Autodesk Inventor part; units mm, degrees
ref_plane "YZ Plane" through (0, 0, 0) normal (1, 0, 0) x (0, 1, 0)
ref_plane "XZ Plane" through (0, 0, 0) normal (0, 1, 0) x (-1, 0, 0)
ref_plane "XY Plane" through (0, 0, 0) normal (0, 0, 1) x (1, 0, 0)
sketch "スケッチ5" plane through (0, 0, 0) normal (1, 0, 0) x (0, 1, 0)
  circle A0 centre (68.5779, -0.3457) radius 120
  line L0 (68.5779, -0.3457) -> (-262.8846, -0.3457) construction
  line L1 (136.0779, -117.2592) -> (-66.4221, -0.3457)
  circle A1 centre (68.5779, -0.3457) radius 5
  line L2 (68.5779, -0.3457) -> (136.0779, 116.5677) construction
  line L3 (68.5779, -0.3457) -> (136.0779, -117.2592) construction
  line L4 (68.5779, -0.3457) -> (-66.4221, -0.3457)
  line L5 (85.6138, 37.1613) -> (80.6138, 28.5011) construction
  line L6 (80.6138, 28.5011) -> (84.0779, 26.5011) construction
  line L7 (84.0779, 26.5011) -> (89.0779, 35.1613) construction
  line L8 (89.0779, 35.1613) -> (85.6138, 37.1613)
  line L9 (89.0779, 35.1613) -> (84.0779, 26.5011) construction
  line L10 (84.0779, 26.5011) -> (87.542, 24.5011) construction
  line L11 (87.542, 24.5011) -> (92.542, 33.1613) construction
  line L12 (92.542, 33.1613) -> (89.0779, 35.1613)
  line L13 (83.1138, 32.8312) -> (90.042, 28.8312) construction
  circle A2 centre (68.5779, -0.3457) radius 2.65 construction
  line L14 (85.3973, 37.2863) -> (78.8973, 26.028) construction
  line L15 (78.8973, 26.028) -> (74.5672, 28.528) construction
  line L16 (74.5672, 28.528) -> (81.0672, 39.7863) construction
  line L17 (81.0672, 39.7863) -> (85.3973, 37.2863)
  line L18 (92.7585, 33.0363) -> (86.2585, 21.778) construction
  line L19 (86.2585, 21.778) -> (90.5886, 19.278) construction
  line L20 (90.5886, 19.278) -> (97.0886, 30.5363) construction
  line L21 (97.0886, 30.5363) -> (92.7585, 33.0363)
  circle A3 centre (68.5779, -0.3457) radius 28.3207 construction
  line L22 (27.5779, 8.9043) -> (27.5779, 3.9043)
  line L23 (27.5779, 3.9043) -> (40.5779, 3.9043) construction
  line L24 (40.5779, 8.9043) -> (27.5779, 8.9043) construction
  line L25 (40.5779, 3.9043) -> (40.5779, 8.9043)
  line L26 (27.5779, -4.5957) -> (40.5779, -4.5957) construction
  line L27 (27.5779, -9.5957) -> (27.5779, -4.5957)
  line L28 (40.5779, -9.5957) -> (27.5779, -9.5957) construction
  line L29 (40.5779, -4.5957) -> (40.5779, -9.5957)
  line L30 (81.0672, -40.4778) -> (85.3973, -37.9778)
  line L31 (85.3973, -37.9778) -> (78.8973, -26.7194) construction
  line L32 (74.5672, -29.2194) -> (81.0672, -40.4778) construction
  line L33 (78.8973, -26.7194) -> (74.5672, -29.2194) construction
  line L34 (92.7585, -33.7278) -> (86.2585, -22.4694) construction
  line L35 (97.0886, -31.2278) -> (92.7585, -33.7278)
  line L36 (90.5886, -19.9694) -> (97.0886, -31.2278) construction
  line L37 (86.2585, -22.4694) -> (90.5886, -19.9694) construction
  line L38 (74.5672, 28.528) -> (73.9509, 27.4606)
  line L39 (90.5886, 19.278) -> (89.9724, 18.2106) construction
  line L40 (40.5779, 8.9043) -> (41.8104, 8.9043)
  line L41 (40.5779, -9.5957) -> (41.8104, -9.5957)
  line L42 (74.5672, -29.2194) -> (70.7713, -22.6449)
  line L43 (90.5886, -19.9694) -> (89.9724, -18.9021) construction
  line L44 (82.1888, 31.229) -> (72.1888, 13.9085) construction
  line L45 (72.1888, 13.9085) -> (66.9926, 16.9085) construction
  line L46 (66.9926, 16.9085) -> (76.9926, 34.229) construction
  line L47 (76.9926, 34.229) -> (82.1888, 31.229)
  circle A4 centre (72.0907, 19.7387) radius 1.5
  circle A5 centre (77.0907, 28.3989) radius 1.5
  circle A6 centre (84.2151, 12.7387) radius 1.5
  circle A7 centre (89.2151, 21.3989) radius 1.5
  circle A8 centre (39.4279, 6.6543) radius 1.5
  circle A9 centre (49.4279, 6.6543) radius 1.5
  circle A10 centre (49.4279, -7.3457) radius 1.5
  circle A11 centre (39.4279, -7.3457) radius 1.5
  circle A12 centre (77.0907, -29.0904) radius 1.5
  circle A13 centre (72.0907, -20.4301) radius 1.5
  circle A14 centre (84.2151, -13.4301) radius 1.5
  circle A15 centre (89.2151, -22.0904) radius 1.5
  line L48 (69.5907, 15.4085) -> (82.1888, 31.229) construction
  circle A16 centre (68.5779, -0.3457) radius 34.3835
  line L49 (60.5779, 46.6543) -> (-119.4221, 46.6543) construction
  line L50 (-119.4221, 46.6543) -> (-119.4221, 31.6543)
  line L51 (-119.4221, 31.6543) -> (60.5779, 31.6543) construction
  line L52 (60.5779, 31.6543) -> (60.5779, 46.6543) construction
  circle A17 centre (50.5779, 39.1543) radius 1.5 construction
  circle A18 centre (40.5779, 39.1543) radius 1.5 construction
  line L53 (34.1944, 46.6543) -> (34.1944, -0.3457) construction
  line L54 (60.5779, 46.6543) -> (87.898, 28.0965) construction
  line L55 (34.1944, -47.3457) -> (34.1944, -0.3457) construction
  line L56 (60.5779, -47.3457) -> (87.898, -28.7879) construction
  line L57 (60.5779, -47.3457) -> (-119.4221, -47.3457) construction
  line L58 (-119.4221, -32.3457) -> (60.5779, -32.3457) construction
  circle A19 centre (40.5779, -39.8457) radius 1.5 construction
  circle A20 centre (50.5779, -39.8457) radius 1.5 construction
  line L59 (68.5779, -0.3457) -> (51.3862, 29.4312)
  line L60 (53.2382, 46.2235) -> (35.9176, 36.2235)
  line L61 (35.9176, 36.2235) -> (40.9176, 27.5632)
  line L62 (40.9176, 27.5632) -> (58.2382, 37.5632)
  line L63 (58.2382, 37.5632) -> (53.2382, 46.2235)
  circle A21 centre (51.408, 39.3934) radius 1.5
  circle A22 centre (42.7478, 34.3934) radius 1.5
  circle A23 centre (42.7478, -35.0848) radius 1.5
  circle A24 centre (51.408, -40.0848) radius 1.5
  circle A25 centre (111.5779, -5.3457) radius 1.5
  circle A26 centre (111.5779, 4.6543) radius 1.5
  circle A27 centre (68.5779, -0.3457) radius 193.5
  line L64 (-124.2868, 15.3208) -> (151.4426, 174.5133)
  line L65 (68.5779, -0.3457) -> (8.5779, 103.5773)
  line L66 (68.5779, -0.3457) -> (68.5779, 193.1543)
  line L67 (117.549, 4.8338) -> (16.049, 180.6369)
  line L68 (16.049, 180.6369) -> (-1.2715, 170.6369)
  line L69 (-1.2715, 170.6369) -> (100.2285, -5.1662)
  line L70 (100.2285, -5.1662) -> (117.549, 4.8338)
  circle A28 centre (37.9737, 117.6622) radius 1.5
  circle A29 centre (13.3039, 170.3917) radius 1.5
  circle A30 centre (58.5779, 16.9748) radius 1.6
  circle A31 centre (68.5779, -0.3457) radius 10 construction
  circle A32 centre (103.8888, 8.494) radius 1.6
  circle A33 centre (93.8888, 25.8145) radius 1.6
  line L71 (117.549, 4.8338) -> (90.6574, -10.6921)
  line L72 (97.549, 39.4748) -> (64.1622, 20.1989)
  line L73 (19.6068, -5.5252) -> (52.9936, 13.7507)
  circle A34 centre (33.267, -9.1855) radius 1.6
  circle A35 centre (43.267, -26.506) radius 1.6
  line L74 (39.6068, -40.1662) -> (-61.8932, 135.6369)
  line L75 (56.9273, -30.1662) -> (39.6068, -40.1662)
  line L76 (39.6068, -40.1662) -> (66.4984, -24.6404)
  line L77 (68.5779, -0.3457) -> (51.3862, -30.1227)
  line L78 (69.2071, -12.256) -> (57.9487, -5.756) construction
  line L79 (57.9487, -5.756) -> (48.9487, -21.3444) construction
  line L80 (48.9487, -21.3444) -> (60.2071, -27.8444) construction
  line L81 (60.2071, -27.8444) -> (69.2071, -12.256) construction
  circle A36 centre (68.5779, -0.3457) radius 28
  circle A37 centre (68.5779, -0.3457) radius 38 construction
  circle A38 centre (68.5779, -0.3457) radius 12.6
  circle A39 centre (58.5779, -17.6662) radius 1.6
  circle A40 centre (88.5779, -0.3457) radius 1.6
  circle A41 centre (66.9902, -26.0957) radius 4
  circle A42 centre (66.9902, -26.0957) radius 1.6
  line L82 (58.2382, 37.5632) -> (60.7896, 33.144)
  line L83 (40.9176, 27.5632) -> (43.4691, 23.144)
  line L84 (58.2382, -38.2547) -> (60.7896, -33.8355)
  line L85 (53.2382, -46.915) -> (58.2382, -38.2547)
  line L86 (35.9176, -36.915) -> (53.2382, -46.915)
  circle A43 centre (51.408, -40.0848) radius 1.5
  circle A44 centre (42.7478, -35.0848) radius 1.5
  line L87 (40.9176, -28.2547) -> (35.9176, -36.915)
  line L88 (40.9176, -28.2547) -> (43.4691, -23.8355)
  line L89 (106.5779, 9.6543) -> (101.4751, 9.6543)
  line L90 (116.5779, 9.6543) -> (106.5779, 9.6543)
  line L91 (116.5779, -10.3457) -> (116.5779, 9.6543)
  circle A45 centre (111.5779, 4.6543) radius 1.5
  circle A46 centre (111.5779, -5.3457) radius 1.5
  line L92 (106.5779, -10.3457) -> (116.5779, -10.3457)
  line L93 (106.5779, -10.3457) -> (101.4751, -10.3457)
  point P0 (0, 0)
  point P1 (53.4487, -13.5502)
  point P2 (44.5779, 41.2235)
  point P3 (44.5779, -41.915)
  point P4 (116.5779, -0.3457)
  point P5 (41.6073, 7.1768)
  point P6 (61.6073, -27.4642)
  point P7 (63.4018, -27.8632)
  point P8 (70.3342, -28.2906)
  point P9 (95.5485, -7.8683)
  point P10 (100.2285, -5.1662)
  point P11 (75.5485, 26.7727)
  dimension "d169" = 3
  dimension "d170" = 3
  dimension "d171" = 10
  dimension "d172" = 10
  dimension "d173" = 7.5
  dimension "d174" = 7.5
  dimension "d175" = 60
  dimension "d176" = 10
  dimension "d177" = 10
  dimension "d178" = 10
  dimension "d179" = 3
  dimension "d180" = 5
  dimension "d181" = 5
  dimension "d182" = 360
  dimension "d183" = 387
  dimension "d184" = 110
  dimension "d185" = 60
  dimension "d186" = 20
  dimension "d187" = 73
  dimension "d188" = 3
  dimension "d189" = 3
  dimension "d190" = 7.5
  dimension "d191" = 7.5
  dimension "d192" = 7.5
  dimension "d193" = 7.5
  dimension "d194" = 3.2
  dimension "d195" = 20
  dimension "d196" = 20
  dimension "d197" = 3.2
  dimension "d198" = 3.2
  dimension "d199" = 10
  dimension "d200" = 10
  dimension "d201" = 10
  dimension "d202" = 20
  dimension "d203" = 10
  dimension "d204" = 120
  dimension "d205" = 13
  dimension "d206" = 18
  dimension "d207" = 6.5
  dimension "d208" = 56
  dimension "d209" = 10
  dimension "d210" = 25.2
  dimension "d211" = 25
  dimension "d212" = 20
  dimension "d213" = 360
  dimension "d214" = 8
  dimension "d215" = 5
  dimension "d216" = 5
  dimension "d217" = 3.2
  dimension "d218" = 360
extrude "押し出し4" add sketch "スケッチ5" against normal blind 2 contours L67 L90 L89 A32 A16 L72 | L67 L91 L70 A16 L89 A32 L90 | A36 L72 L66 | L66 A38 L59 A30 A36 | L67 L70 L91 | A16 L70 L69 A36 L72 | L73 A16 L4 | L4 A16 L88 A35 L87 L74 L73 | L69 A36 L72 A5 | L72 A36 L69 A41 L76 L77 A39 A38 L66 | L59 A30 A38 L4 A36 | A16 L73 A8 A36 L4 | L4 A36 L77 A16 | L87 L88 A35 A16 L75 L86 L74 | A36 L69 | A5 L72 | A38 L77 A1 L66 | L66 A1 L59 A38 | L4 A38 L77 A39 A36 | L73 L25 A8 | L86 L75 L74 | L69 L71 A36 | L59 A1 L4 A38 | A8 L25 L73 | L4 A1 L77 A38 | A36 L76 L75 A16 L77 | A39 L77 | L77 A39 | L76 A41 A36 | A41 A36 | A36 A41 | A11 L29 | L29 A11 | A4 | A6 | A7 | A9 | A10 | A13 | A14 | A23 | A26 picked at (77.6802, 27.4001) picked at (39.3486, 5.7524) picked at (40.6415, 6.0852)
extrude "押し出し5" cut sketch "スケッチ5" against normal blind 2 contours A38 L77 A1 L66 | L66 A1 L59 A38 | L59 A1 L4 A38 | L4 A1 L77 A38
fillet "フィレット4" radius 2 10 edges at (-1, 95.5485, -7.8683) (-1, 117.549, 4.8338) (-1, 97.549, 39.4748) (-1, 75.5485, 26.7727) (-1, 41.6073, 7.1768) (-1, 19.6068, -5.5252) (-1, 39.6068, -40.1662) (-1, 61.6073, -27.4642) (-1, 63.4018, -27.8632) (-1, 70.3342, -28.2906)
equation "\"d174\" = d173"
equation "\"d200\" = d201"
properties part number "hand-grab-v3-Plate-ASP_F" material "アルミニウム 6061"
Can you work these out from the model? Positions are in its coordinate system, mm. Round coordinates to 2 decimals unless told otherwise and drop trailing zeros. Order: outer loops, then holes, each group sorted by start corner. A loop starts at its lowest first (then second) coordinate and runs counter-clockwise, first axis right, second up. Notation, with made-up numbers: M 59.25,-29.5 L 78.25,-29.5 A26 cw 78.25,3.5 Z; hole C 21,-6 d2. An arc over 180 degrees is marked long. Use a Markdown table: item, result.
1) Imagine slicing it at D-D (z = 32.5). List the corners of the cut face in (x, y) for me.
Geometry says:
| item | result |
|---|---|
| outline | M -2,85.47 L 0,85.47 L 0,101.58 L -2,101.58 Z |
2) I'm going to push a flat-ended pin straight in: P1, Ø2.5, axis at y = 103.89, z = 8.49, coming from the -X side. Where does the tip first touch, or does it pass through?
Geometry says:
| item | result |
|---|---|
| P1 | passes through |
3) Imagine slicing it at A-A (y = 73.5). List the corners of the cut face in (x, z) for me, then the cut area to 3 significant figures.
Geometry says:
| item | result |
|---|---|
| outline | M -2,-27.91 L 0,-27.91 L 0,-11.94 L -2,-11.94 Z; M -2,11.25 L 0,11.25 L 0,27.22 L -2,27.22 Z |
| area | 63.9 mm² |
4) Imagine slicing it at B-B (x = -1.45). Give the number of separate pieces and of enclosed holes in the cut face, then the cut area to 3 significant figures.
Geometry says:
| item | result |
|---|---|
| separate pieces | 1 |
| enclosed holes | 8 |
| area | 3,480 mm² |
5) If I drill on line 1 along Y through (x, z) = (-1.5, 1); line 2 along Y through (x, z) = (-1.35, 9); line 3 along Y through (x, z) = (-1.5, 17), over which ranges is the centre line in solid material (lowest first)?
Geometry says:
| item | result |
|---|---|
| line 1 | y = 30.91 to 56.05, 81.11 to 87.71, 89.44 to 110.91 |
| line 2 | y = 42.18 to 60.13, 77.03 to 102.37, 105.41 to 115.14 |
| line 3 | y = 46.6 to 56.98, 60.18 to 110.52 |
6) If we mould it in two halves opening along Y, with no side actions, what happens to faces 1 (the face through (-0.986, 66.695, -30.085)), 2 (the face through (-0.986, 86.045, -22.23)), 3 (the face through (0, 79, -8))? For each: +Y half, -Y half, draft (parallel to the pull), parting line (faces both ways), or undercut.
Geometry says:
| item | result |
|---|---|
| face 1 | undercut |
| face 2 | +Y half |
| face 3 | draft |
7) Imagine slicing it at C-C (y = 94). List the corners of the cut face in (x, z) for me.
Geometry says:
| item | result |
|---|---|
| outline | M -2,-12.08 L 0,-12.08 L 0,24.22 L -2,24.22 Z; M -2,27.41 L 0,27.41 L 0,37.43 L -2,37.43 Z |
